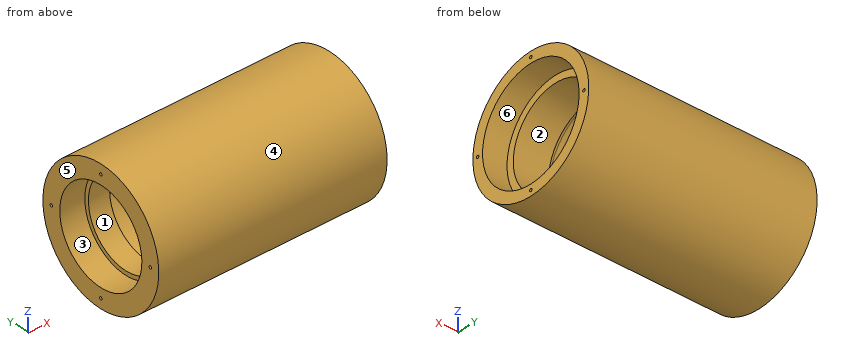
```python
from build123d import *

# Parameters (mm, degrees)
BOSS_EXTRUDE1_DEPTH          = 84
BOSS_EXTRUDE1_DEPTH_BACK     = 84
SKETCH2_R                    = 48
CUT_EXTRUDE1_DEPTH           = 40
CUT_EXTRUDE1_DEPTH_BACK      = 50
SKETCH3_R                    = 40
CUT_EXTRUDE2_DEPTH           = 109
CUT_EXTRUDE2_DEPTH_BACK      = 109
SKETCH4_R                    = 31
FILLET1_R                    = 5
CUT_EXTRUDE3_REACH           = 176
CUT_EXTRUDE3_START           = -66
SKETCH5_R                    = 40
SKETCH6_R                    = 34
CUT_EXTRUDE4_DEPTH           = 18.4
M2_5X0_45_TAPPED_HOLE1_D     = 2.05
M2_5X0_45_TAPPED_HOLE1_DEPTH = 8
M2_5X0_45_TAPPED_HOLE1_TIP   = 0.615882135
M2_5X0_45_TAPPED_HOLE2_D     = 2.05
M2_5X0_45_TAPPED_HOLE2_DEPTH = 8
M2_5X0_45_TAPPED_HOLE2_TIP   = 0.615882135
CUT_EXTRUDE6_START           = -18
SKETCH14_R                   = 34.825
CUT_EXTRUDE6_DEPTH           = 26


with BuildPart() as part:
    # Sketch2 → Boss-Extrude1 (new, two sides: drawn at the far end of the back side and taken through both)
    with BuildSketch(Plane(origin=(0, 0, 0), x_dir=(0, -1, 0), z_dir=(1, 0, 0)).offset(-BOSS_EXTRUDE1_DEPTH_BACK)):
        with Locations(Location((0, 0, 0), (0, 0, 90))):
            Circle(SKETCH2_R)
    extrude(amount=BOSS_EXTRUDE1_DEPTH + BOSS_EXTRUDE1_DEPTH_BACK)

    # Sketch3 → Cut-Extrude1 (cut, two sides: drawn at the far end of the back side and taken through both)
    with BuildSketch(Plane(origin=(0, 0, 0), x_dir=(0, -1, 0), z_dir=(1, 0, 0)).offset(-CUT_EXTRUDE1_DEPTH_BACK)):
        with Locations(Location((0, 0, 0), (0, 0, 90))):
            Circle(SKETCH3_R)
    extrude(amount=CUT_EXTRUDE1_DEPTH + CUT_EXTRUDE1_DEPTH_BACK, mode=Mode.SUBTRACT)

    # Sketch4 → Cut-Extrude2 (cut, two sides: drawn at the far end of the back side and taken through both)
    with BuildSketch(Plane(origin=(0, 0, 0), x_dir=(0, -1, 0), z_dir=(1, 0, 0)).offset(-CUT_EXTRUDE2_DEPTH_BACK)):
        with Locations(Location((0, 0, 0), (0, 0, 90))):
            Circle(SKETCH4_R)
    extrude(amount=CUT_EXTRUDE2_DEPTH + CUT_EXTRUDE2_DEPTH_BACK, mode=Mode.SUBTRACT)

    # Fillet1
    fillet1_edges = [part.edges().sort_by_distance(p)[0] for p in [
        (40, 0, 40),
        (-50, 0, 40),
    ]]
    fillet(fillet1_edges, radius=FILLET1_R)

    # Sketch5 → Cut-Extrude3 (cut, up to next)
    with BuildSketch(Plane(origin=(0, 0, 0), x_dir=(0, 0, -1), z_dir=(-1, 0, 0)).offset(CUT_EXTRUDE3_START), mode=Mode.PRIVATE) as cut_extrude3_sk1:
        Circle(SKETCH5_R)
    cut_extrude3_tool1 = extrude(cut_extrude3_sk1.sketch, amount=-CUT_EXTRUDE3_REACH, mode=Mode.PRIVATE) & part.part
    add(cut_extrude3_tool1.solids().sort_by_distance((66, 0, 0))[0], mode=Mode.SUBTRACT)

    # Sketch6 → Cut-Extrude4 (cut)
    with BuildSketch(Plane.ZY.offset(84)):
        Circle(SKETCH6_R)
    extrude(amount=-CUT_EXTRUDE4_DEPTH, mode=Mode.SUBTRACT)

    # M2.5x0.45 Tapped Hole1
    with Locations(Plane(origin=(84, 0, 0), x_dir=(0, 0, -1), z_dir=(1, 0, 0))):
        with Locations((256.353874164, 80.103153953), (0, -44), (-44, 0), (0, 44), (44, 0)):
            Hole(M2_5X0_45_TAPPED_HOLE1_D / 2, depth=M2_5X0_45_TAPPED_HOLE1_DEPTH)
            with Locations((0, 0, -(M2_5X0_45_TAPPED_HOLE1_DEPTH + M2_5X0_45_TAPPED_HOLE1_TIP / 2))):  # 118° drill point
                Cone(0, M2_5X0_45_TAPPED_HOLE1_D / 2, M2_5X0_45_TAPPED_HOLE1_TIP, mode=Mode.SUBTRACT)

    # M2.5x0.45 Tapped Hole2
    with Locations(Plane.ZY.offset(84)):
        with Locations((0, 41), (0, -41), (41, 0), (-41, 0)):
            Hole(M2_5X0_45_TAPPED_HOLE2_D / 2, depth=M2_5X0_45_TAPPED_HOLE2_DEPTH)
            with Locations((0, 0, -(M2_5X0_45_TAPPED_HOLE2_DEPTH + M2_5X0_45_TAPPED_HOLE2_TIP / 2))):  # 118° drill point
                Cone(0, M2_5X0_45_TAPPED_HOLE2_D / 2, M2_5X0_45_TAPPED_HOLE2_TIP, mode=Mode.SUBTRACT)

    # Sketch14 → Cut-Extrude6 (cut)
    with BuildSketch(Plane(origin=(84, 0, 0), x_dir=(0, 0, -1), z_dir=(1, 0, 0)).offset(CUT_EXTRUDE6_START)):
        Circle(SKETCH14_R)
    extrude(amount=-CUT_EXTRUDE6_DEPTH, mode=Mode.SUBTRACT)


solid = part.part
```
CAD build for the part. Positions are in the model's coordinates, mm. Face numbers are marked on the shaded views. A direction names the side the tool comes from. Round coordinates to 2 decimals unless told otherwise and drop trailing zeros. Write each loop counter-clockwise with the first axis right and the second up, starting at its lowest first coordinate (ties: lowest second). Pieces come first, ordered by that corner, then holes. Notation, with made-up numbers: M 50.5,16.25 L 89.5,16.25 A20 cw 89.5,54.25 Z; hole C 16,-20.75 d11. An arc over 180 degrees is marked long. One line per question, with ' | ' between items.
1. Mould opens along Z. For the marked faces 3, 4, 5 and 6 say: pulls with the +Z half, pulls with the -Z half, needs draft (parallel to the pull), parting line crosses it, or undercut.
Working result:
face 3: undercut | face 4: parting line crosses it | face 5: needs draft | face 6: undercut
2. Pin check, flat tips, straight feed: pin 1 Ø3 at (x, z) = (-1.5, 15) entering from +Y; pin 2 Ø1.5 at (x, y) = (57, -10) entering from -Z; pin 3 Ø2 at (x, z) = (-17, -32) entering from -Y. Stop position of each tip, or through.
Working result:
pin 1: y = 46.06 | pin 2: z = -47.1 | pin 3: y = -36.65
3. Cut at A-A on x = 60.5. Write the cut outline in (y, z) (3 decimals), and give its area (3 significant figures).
Working result:
outline: C 0,0 d96; hole C 0,0 d69.65 | area: 3,430 mm2
4. Which spindle directions (+Z, -Z, +X, -X, +Y, -Y) get a long thin tool onto all of the face, cutting with end or side? Do the marked faces 1 and 2. Say none if no direction does.
Working result:
face 1: +X, -X | face 2: +X
5. Cut at B-B on x = -37.5. Write the cut outline in (y, z).
Working result:
outline: C 0,0 d96; hole C 0,0 d80
6. Probe L1, parallel to Y at x = 78.5, z = 0 (3 decimals); L2, parallel to Y at x = 47, z = -1; L3, parallel to Y at x = -76, z = 0 (3 decimals). List the from-to ranges inside material, lowest first. Write a range as from..to.
Working result:
L1: -48..-45.025, -42.975..-40, 40..42.975, 45.025..48 | L2: -47.99..-34.81, 34.81..47.99 | L3: -48..-42.025, -39.975..-34, 34..39.975, 42.025..48
